Input: dimensioned drawing with shaded views. Units: mm. Origin: part minimum x, y, z. Give positions to 0.01 mm unless a question says otherwise; leave off trailing zeros. Order: outer loops, then holes, each group sorted by start corner. A loop starts at its lowest first (then second) coordinate and runs counter-clockwise, first axis right, second up. Notation, with made-up numbers: (23.5, 63) - (38.5, 63) arc R21 ccw to (38.5, 98) - close; hole circle Ø1 at (66.5, 16.5). An arc over 180 degrees is marked (long way). Use a Markdown table: item, result.
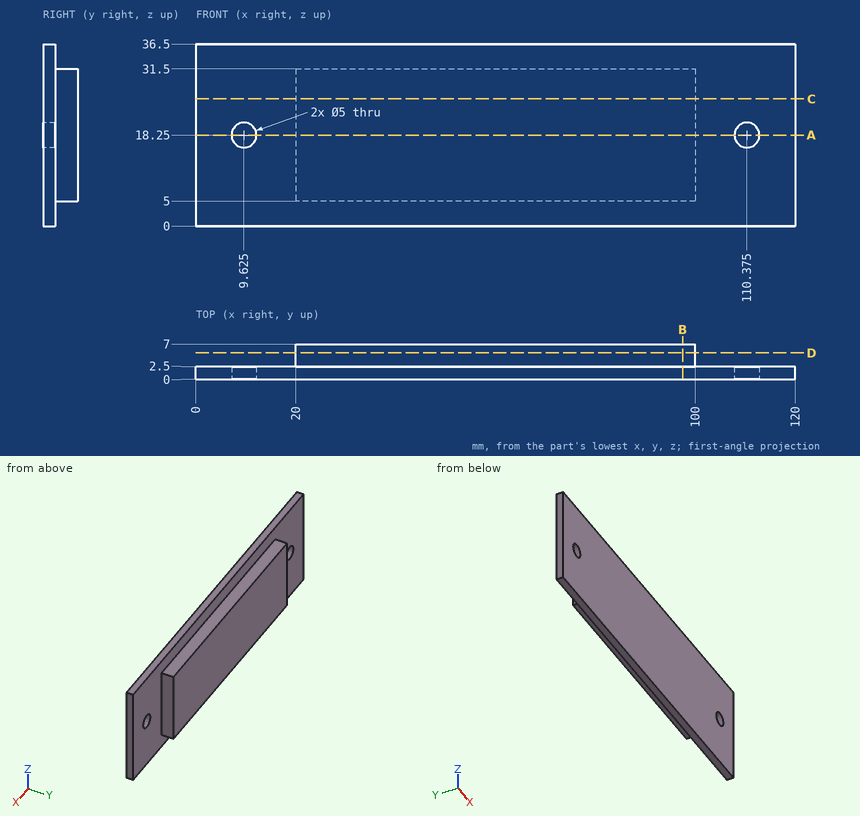
1. Section query C-C (z = 25.5). Return loops of the section in (x, y), then the cut area to 3 significant figures.
Response:
| item | result |
|---|---|
| outline | (0, 0) - (120, 0) - (120, 2.5) - (100, 2.5) - (100, 7) - (20, 7) - (20, 2.5) - (0, 2.5) - close |
| area | 660 mm^2 |
2. Section query D-D (y = 5.25). Return loops of the section in (x, z).
Response:
| item | result |
|---|---|
| outline | (20, 5) - (100, 5) - (100, 31.5) - (20, 31.5) - close |
3. Material intervals for line 1 along X through (y, z) = (1.8, 18.25) (3 decimals); line 2 along X through (y, z) = (3.25, 12); line 3 along Z through (x, y) = (78.5, 3.25), sorted ascending.
Response:
| item | result |
|---|---|
| line 1 | x = 0 to 7.125, 12.125 to 107.875, 112.875 to 120 |
| line 2 | x = 20 to 100 |
| line 3 | z = 5 to 31.5 |
4. Pin query (flat end, axial travel): pin 1 (1.3 mm diameter, centred on x = 48, y = 4.5, fed in from -Z); pin 2 (3.5 mm diameter, centred on y = 5.5, z = 23.5, fed in from -X); pin 3 (1.3 mm diameter, centred on x = 42.5, y = 4.5, fed in from +Z). Return the tip coordinate at first contact, or that it passes through.
Response:
| item | result |
|---|---|
| pin 1 | stops at z = 5 |
| pin 2 | stops at x = 20 |
| pin 3 | stops at z = 31.5 |
5. Section query B-B (x = 97.5). Return loops of the section in (y, z).
Response:
| item | result |
|---|---|
| outline | (0, 0) - (2.5, 0) - (2.5, 5) - (7, 5) - (7, 31.5) - (2.5, 31.5) - (2.5, 36.5) - (0, 36.5) - close |
6. Section query A-A (z = 18.25). Return loops of the section in (x, y) (3 decimals).
Response:
| item | result |
|---|---|
| outline | (0, 0) - (7.125, 0) - (7.125, 2.5) - (0, 2.5) - close; (12.125, 0) - (107.875, 0) - (107.875, 2.5) - (100, 2.5) - (100, 7) - (20, 7) - (20, 2.5) - (12.125, 2.5) - close; (112.875, 0) - (120, 0) - (120, 2.5) - (112.875, 2.5) - close |
